Geometry check sheet. Reference: drawing and pictorial views, mm from the part's lowest x, y, z. A direction names the side the tool comes from. Round coordinates to 2 decimals unless told otherwise and drop trailing zeros. Write each loop counter-clockwise with the first axis right and the second up, starting at its lowest first coordinate (ties: lowest second). Pieces come first, ordered by that corner, then holes. Notation, with made-up numbers: M 27.25,64 L 82.25,64 A19 ccw 82.25,99 Z; hole C 83.25,-25 d1. An arc over 180 degrees is marked long. One line per question, with ' | ' between items.
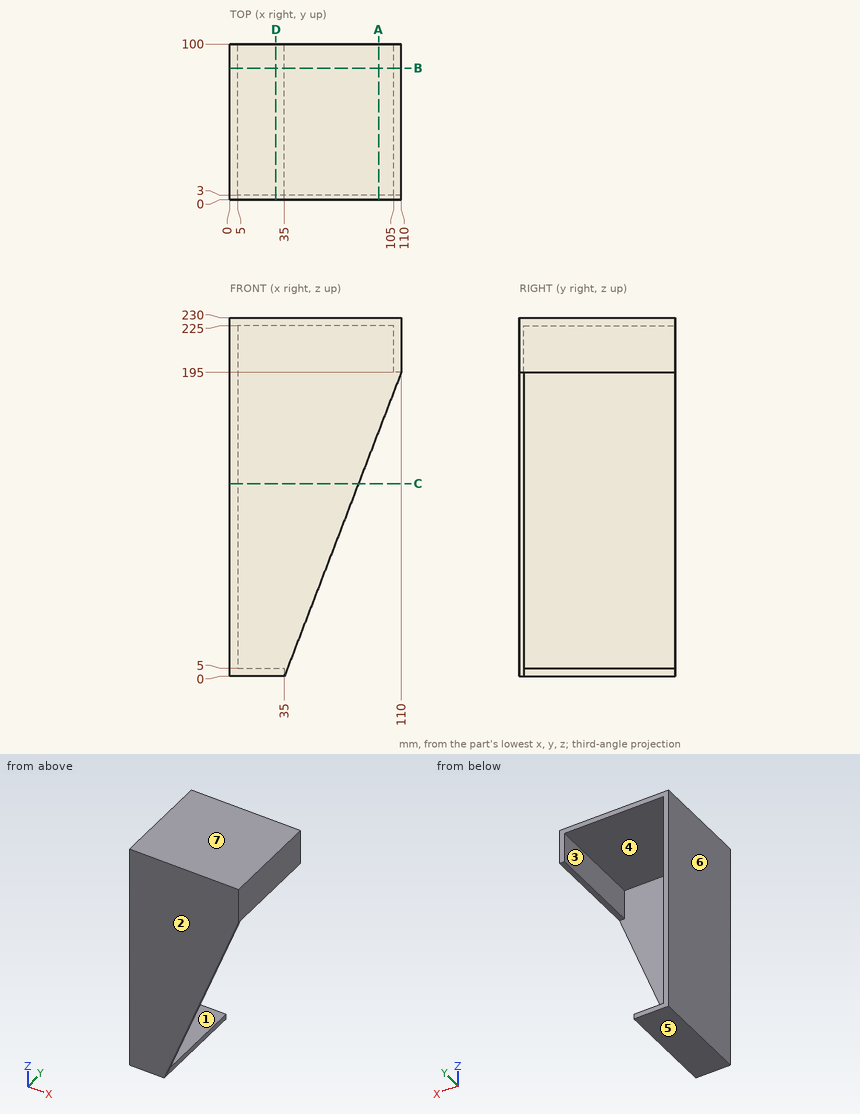
1. Go/stop test with flat-tipped pins: P1, Ø2.5, axis at x = 108, y = 28.5, coming from the -Z side; P2, Ø4, axis at y = 48.5, z = 1.5, coming from the +X side; P3, Ø10, axis at x = 42, z = 42.5, coming from the +Y side. Record where each tip stops, or that it passes through.
Results:
P1: stops at z = 195 | P2: stops at x = 35 | P3: stops at y = 3
2. Section check B-B, the plane y = 84.5. Record the cut outline in (x, z).
Results:
outline: M 0,0 L 35,0 L 35,5 L 5,5 L 5,225 L 105,225 L 105,195 L 110,195 L 110,230 L 0,230 Z
3. Section check D-D, the plane x = 29.5. Record the cut outline in (y, z), then the cut area to 3 significant figures.
Results:
outline: M 0,0 L 100,0 L 100,5 L 3,5 L 3,225 L 100,225 L 100,230 L 0,230 Z | area: 1,660 mm2
4. Mould release check, pull along Z, two halves, no side actions. Record for the marked faces 4, 5, 6 and 7: pulls with the +Z half, pulls with the -Z half, needs draft (parallel to the pull), parting line crosses it, or undercut.
Results:
face 4: undercut | face 5: pulls with the -Z half | face 6: needs draft | face 7: pulls with the +Z half
5. Section check A-A, the plane x = 95.5. Record the cut outline in (y, z), then the cut area to 3 significant figures.
Results:
outline: M 0,157.3 L 3,157.3 L 3,225 L 100,225 L 100,230 L 0,230 Z | area: 703 mm2
6. Tool access check on the marked faces 1, 2 and 3. Record the directions out of +Z, -Z, +X, -X, +Y, -Y that give a thin tool (end or side, any length) a straight path to the whole face; none if there is none.
Results:
face 1: +X, +Y | face 2: +Z, -Z, +X, -X, -Y | face 3: -Z, +Y
7. Section check C-C, the plane z = 123.5. Record the cut outline in (x, y).
Results:
outline: M 0,0 L 82.5,0 L 82.5,3 L 5,3 L 5,100 L 0,100 Z
8. Thickness scan on line 1 (Z direction, x = 13, y = 30); line 2 (X direction, y = 68.5, z = 207); line 3 (Y direction, x = 77.5, z = 163). Record the ranges inside material, lowest first.
Results:
line 1: z = 0 to 5, 225 to 230 | line 2: x = 0 to 5, 105 to 110 | line 3: y = 0 to 3
